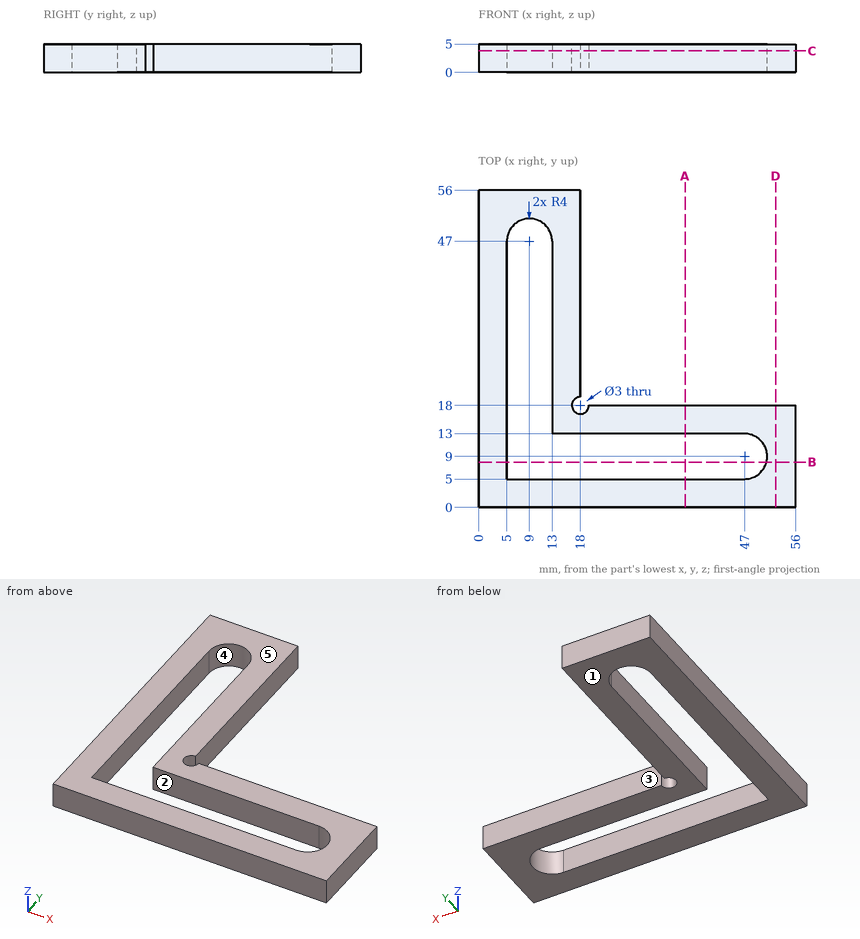
Source: three-view drawing plus pictorial views. Frame: mm from the lowest corner of the part. A direction names the side the tool comes from. Coordinates: 2 decimals unless noted, no trailing zeros. Order: outer loops, then holes, each group sorted by start corner. A loop starts at its lowest first (then second) coordinate and runs counter-clockwise, first axis right, second up.
1) First-contact query: P1, Ø2.5, axis at y = 28.5, z = 2.5, coming from the +X side; P2, Ø1.5, axis at x = 47.5, z = 1.5, coming from the +Y side. Flat tips, straight axial feed; report the tip coordinate or a pass-through.
Result sheet:
P1: stops at x = 18
P2: stops at y = 18
2) Section A-A (x = 36.5). Return loops of the section in (y, z).
Result sheet:
outline: (0, 0) - (5, 0) - (5, 5) - (0, 5) - close; (13, 0) - (18, 0) - (18, 5) - (13, 5) - close
3) Ray query, probe 1 along X at (y, z) = (26, 3.75); probe 2 along X at (y, z) = (13.5, 3.1). Return the intervals inside material, ascending.
Result sheet:
probe 1: x = 0 to 5, 13 to 18
probe 2: x = 0 to 5, 13 to 56
4) Section D-D (x = 52.5). Return loops of the section in (y, z).
Result sheet:
outline: (0, 0) - (18, 0) - (18, 5) - (0, 5) - close
5) Set-up query: the marked faces 3, 4 and 5. Return all of +Z, -Z, +X, -X, +Y, -Y with unobstructed straight access to the full face (end or side cutting, diameter ignored); none if empty.
Result sheet:
face 3: +Z, -Z, +X, +Y
face 4: +Z, -Z
face 5: +Z, +X, -X, +Y, -Y
6) Section B-B (y = 8). Return loops of the section in (x, z), then the cut area to 3 significant figures.
Result sheet:
outline: (0, 0) - (5, 0) - (5, 5) - (0, 5) - close; (50.87, 0) - (56, 0) - (56, 5) - (50.87, 5) - close
area: 50.6 mm2
7) Section C-C (z = 3.8). Return loops of the section in (x, y).
Result sheet:
outline: (0, 0) - (56, 0) - (56, 18) - (19.5, 18) arc R1.5 cw (long way) to (18, 19.5) - (18, 56) - (0, 56) - close; hole (5, 5) - (47, 5) arc R4 ccw to (47, 13) - (13, 13) - (13, 47) arc R4 ccw to (5, 47) - close
8) Draft query along X for the marked faces 1 and 2. Return one class per face: released by +X, released by -X, zero draft, split by the parting line, or undercut.
Result sheet:
face 1: zero draft
face 2: undercut
